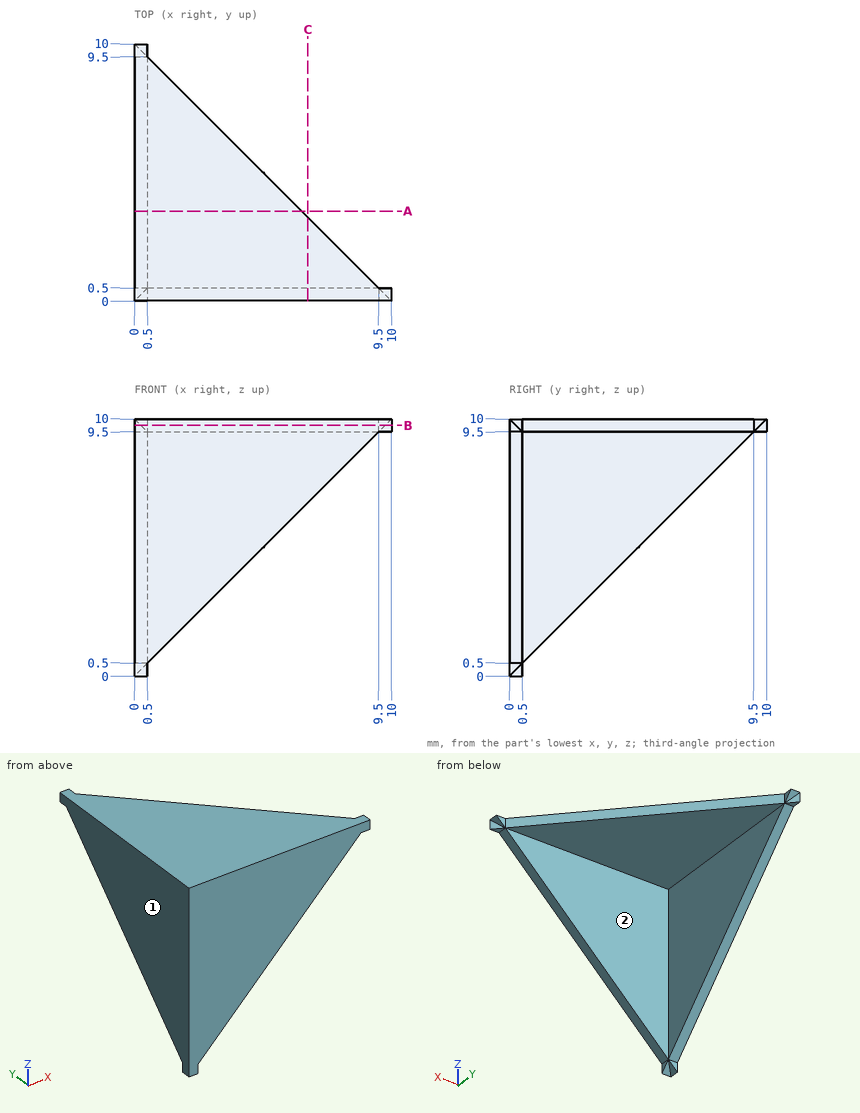
Source: three-view drawing plus pictorial views. Frame: mm from the lowest corner of the part. A direction names the side the tool comes from. Round coordinates to 2 decimals unless told otherwise and drop trailing zeros. Write each loop counter-clockwise with the first axis right and the second up, starting at its lowest first coordinate (ties: lowest second). Pieces come first, ordered by that corner, then holes. Notation, with made-up numbers: M 58.25,65.5 L 108.25,65.5 A18 cw 108.25,92.5 Z; hole C 8,31 d2. An arc over 180 degrees is marked long. One line per item, written item: value. Start each with the question number.
Item 1: Ray query, L1, parallel to X at y = 2.75, z = 8.75; L2, parallel to Z at x = 7.25, y = 1.75. Return the intervals inside material, ascending. Write a range as from..to.
Item 2: Section query A-A (y = 3.5). Return the cut outline in (x, z), plus the area to 3 significant figures.
Item 3: Set-up query: the marked faces 1 and 2. Return all of +Z, -Z, +X, -X, +Y, -Y with unobstructed straight access to the full face (end or side cutting, diameter ignored); none if empty.
Item 4: Section query C-C (x = 6.75). Return the cut outline in (y, z), plus the area to 3 significant figures.
Item 5: Section query B-B (z = 9.75). Return the cut outline in (x, y), plus the area to 3 significant figures.
Item 6: Pin query (flat end, axial travel): pin 1 (2.5 mm diameter, centred on x = 4, y = 3, fed in from -Z); pin 2 (0.6 mm diameter, centred on x = 0.5, z = 0, fed in from +Y); pin 3 (5 mm diameter, centred on y = 6.5, z = 1, fed in from -X). Return the tip coordinate at first contact, or that it passes through.
Result set:
1. L1: x = 0..0.5
1. L2: z = 9.5..10
2. outline: M 0,3.5 L 0.5,3.5 L 0.5,9.5 L 6.5,9.5 L 6.5,10 L 0,10 Z
2. area: 6.25 mm²
3. face 1: +Z, -Z, -X, +Y, -Y
3. face 2: -Z, +X, +Y
4. outline: M 0,6.75 L 0.5,6.75 L 0.5,9.5 L 3.25,9.5 L 3.25,10 L 0,10 Z
4. area: 3.00 mm²
5. outline: M 0,0 L 10,0 L 9.75,0.25 L 9.75,0.5 L 9.5,0.5 L 0.5,9.5 L 0.5,9.75 L 0.25,9.75 L 0,10 Z
5. area: 50.1 mm²
6. pin 1: stops at z = 9.5
6. pin 2: stops at y = 0.3
6. pin 3: passes through
